Design review of the part built by this model. Coordinates are the model's own, in mm. Face numbers are marked on the shaded views. A direction names the side the tool comes from. Give positions to 0.01 mm unless a question says otherwise; leave off trailing zeros. Loops run counter-clockwise (first coordinate to the right, second up) from the corner with the lowest first, then second, coordinate; pieces in that order, holes last. Notation, with made-up numbers: (-15.75, 59) -> (1.25, 59) arc R25 cw to (1.25, 82) -> close; hole circle Ø4 at (67.5, 23). An arc over 180 degrees is marked (long way). Use a Markdown table: item, result. Add a question column.
1. To check wall thickness, follow line 1 (Y direction, x = -2, z = 0); line 2 (Y direction, x = -14.5, z = 0); line 3 (Z direction, x = -3, y = -1.5). State the ranges of each line that lie inside material, in increasing order.
2. Add section A-A (z = 0). State the section outline as (x, y) points.
3. For pin 1 Ø5 at (x, z) = (-17.5, 1.5) entering from +Y; pin 2 Ø10 at (x, y) = (-13.5, -25) entering from -Z; pin 3 Ø4 at (x, z) = (-19, 22) entering from +Y, all flat-tipped, find the tip position at first contact; note any pin that passes through.
4. For the marked faces 5, 6 and 7, list the 3-axis set-ups (+Z, -Z, +X, -X, +Y, -Y) from which the entire face can be reached by the end or side of a thin tool; tool diameter is ignored.
5. Add section D-D (y = 11). State the section outline as (x, z) points, and give its area (3 significant figures).
6. Draft analysis for pull direction Z (two halves, no side actions). For the marked faces 1, 2, 3 and 4, state which applies: pulls with the +Z half, pulls with the -Z half, needs draft (parallel to the pull), parting line crosses it, or undercut.
```python
from build123d import *

# Parameters (mm, degrees)
CUT_EXTRUDE6_DEPTH = 65.031242374
CIRPATTERN6_COUNT  = 8


with BuildPart() as part:
    # Sketch2 → Revolve1 (revolve)
    with BuildSketch(Plane.XY, mode=Mode.PRIVATE) as revolve1_sk:
        Polygon((0, 5), (-30, 5), (-30, 10), (-25, 10), (-25, 15), (-30, 15), (-30, 40), (0, 40), (0, 15), (-5, 15), (-5, 10), (0, 10), align=None)
    revolve(revolve1_sk.sketch.rotate(Axis((0, 0, 0), (-1, 0, 0)), 90), axis=Axis((0, 0, 0), (-1, 0, 0)))

    # Sketch8 → Cut-Extrude6 (cut, through all)
    with BuildSketch(Plane.ZY.offset(30)):
        Polygon((-10, 45), (10, 45), (5, 19), (-5, 19), align=None)
    cut_extrude6 = extrude(amount=-CUT_EXTRUDE6_DEPTH, mode=Mode.SUBTRACT)

    # CirPattern6: Cut-Extrude6 ×8 about axis
    cirpattern6_axis = Axis((0, 0, 0), (1, 0, 0))
    for i in range(1, CIRPATTERN6_COUNT):
        add(cut_extrude6.rotate(cirpattern6_axis, i * 360 / CIRPATTERN6_COUNT), mode=Mode.SUBTRACT)


solid = part.part
```
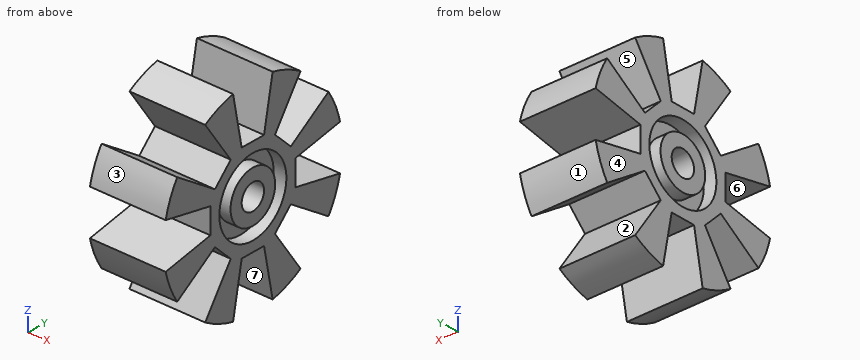
Taken from the geometry:
| question | item | result |
|---|---|---|
| 1 | line 1 | y = -19 to -15, -10 to -5, 5 to 10, 15 to 19 |
| 1 | line 2 | y = -19 to -5, 5 to 19 |
| 1 | line 3 | z = -19 to -14.92, -9.89 to -4.77, 4.77 to 9.89, 14.92 to 19 |
| 2 | outline | (-30, -19) -> (0, -19) -> (0, -15) -> (-5, -15) -> (-5, -10) -> (0, -10) -> (0, -5) -> (-30, -5) -> (-30, -10) -> (-25, -10) -> (-25, -15) -> (-30, -15) -> close; (-30, 5) -> (0, 5) -> (0, 10) -> (-5, 10) -> (-5, 15) -> (0, 15) -> (0, 19) -> (-30, 19) -> (-30, 15) -> (-25, 15) -> (-25, 10) -> (-30, 10) -> close |
| 3 | pin 1 | stops at y = 19 |
| 3 | pin 2 | stops at z = -34.64 |
| 3 | pin 3 | stops at y = 34.64 |
| 4 | face 5 | +X, -X |
| 4 | face 6 | +X, -X, -Y |
| 4 | face 7 | -Z, +X, -X |
| 5 | outline | (-30, -38.46) -> (0, -38.46) -> (0, -18.6) -> (-30, -18.6) -> close; (-30, -15.87) -> (0, -15.87) -> (0, -10.2) -> (-5, -10.2) -> (-5, 10.2) -> (0, 10.2) -> (0, 15.87) -> (-30, 15.87) -> (-30, 10.2) -> (-25, 10.2) -> (-25, -10.2) -> (-30, -10.2) -> close; (-30, 18.6) -> (0, 18.6) -> (0, 38.46) -> (-30, 38.46) -> close |
| 5 | area | 1,940 mm^2 |
| 6 | face 1 | pulls with the -Z half |
| 6 | face 2 | undercut |
| 6 | face 3 | pulls with the +Z half |
| 6 | face 4 | needs draft |
